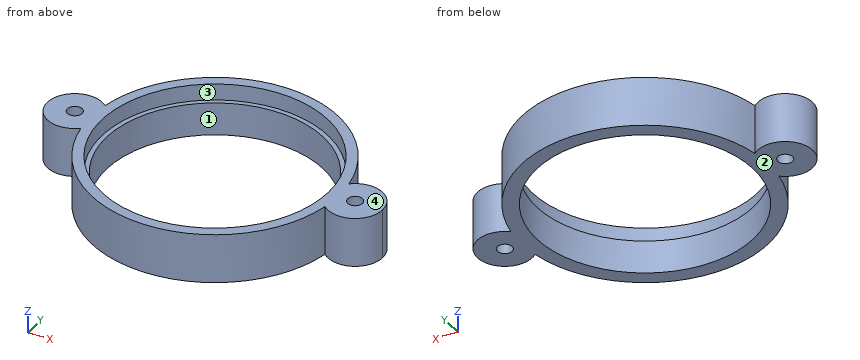
```python
from build123d import *

# Parameters (mm, degrees)
F0_R     = 1.35
F1_DEPTH = 9
F0_R_2   = 19.75
F2_DEPTH = 6
F3_R     = 22.5
F3_R_2   = 20.6
F4_DEPTH = 3


with BuildPart() as f1:
    # F0 (on Top) → F1 (new body)
    with BuildSketch(Plane.XY):
        with BuildLine():
            ThreePointArc((-22.1862745098, -3.7442253372), (-22.5, 0), (-22.1862745098, 3.7442253372))
            ThreePointArc((-22.1862745098, 3.7442253372), (-30.5, 0), (-22.1862745098, -3.7442253372))
        make_face()
        with Locations((-25.5, 0)):
            Circle(F0_R, mode=Mode.SUBTRACT)
    extrude(amount=F1_DEPTH)



with BuildPart() as f1b:
    # F0 (on Top) → F1, piece 2 (new body)
    with BuildSketch(Plane.XY):
        with BuildLine():
            ThreePointArc((22.1862745098, 3.7442253372), (22.4214314493, 1.8786728733), (22.5, 0))
            ThreePointArc((22.5, 0), (22.4214314493, -1.8786728733), (22.1862745098, -3.7442253372))
            ThreePointArc((22.1862745098, -3.7442253372), (27.5532136456, -4.5589816544), (30.5, 0))
            ThreePointArc((30.5, 0), (27.5532136456, 4.5589816544), (22.1862745098, 3.7442253372))
        make_face()
        with Locations((25.5, 0)):
            Circle(F0_R, mode=Mode.SUBTRACT)
    extrude(amount=F1_DEPTH)


with BuildPart() as f2:
    # F0 (on Top) → F2 (new body)
    with BuildSketch(Plane.XY):
        with BuildLine():
            ThreePointArc((22.1862745098, -3.7442253372), (20.5, 0), (22.1862745098, 3.7442253372))
            ThreePointArc((22.1862745098, 3.7442253372), (0, 22.5), (-22.1862745098, 3.7442253372))
            ThreePointArc((-22.1862745098, 3.7442253372), (-20.9410183456, 2.0532136456), (-20.5, 0))
            ThreePointArc((-20.5, 0), (-20.9410183456, -2.0532136456), (-22.1862745098, -3.7442253372))
            ThreePointArc((-22.1862745098, -3.7442253372), (0, -22.5), (22.1862745098, -3.7442253372))
        make_face()
        Circle(F0_R_2, mode=Mode.SUBTRACT)
        with BuildLine():
            ThreePointArc((22.1862745098, -3.7442253372), (22.4214314493, -1.8786728733), (22.5, 0))
            ThreePointArc((22.5, 0), (22.4214314493, 1.8786728733), (22.1862745098, 3.7442253372))
            ThreePointArc((22.1862745098, 3.7442253372), (20.5, 0), (22.1862745098, -3.7442253372))
        make_face()
        with BuildLine():
            ThreePointArc((-20.5, 0), (-20.9410183456, 2.0532136456), (-22.1862745098, 3.7442253372))
            ThreePointArc((-22.1862745098, 3.7442253372), (-22.5, 0), (-22.1862745098, -3.7442253372))
            ThreePointArc((-22.1862745098, -3.7442253372), (-20.9410183456, -2.0532136456), (-20.5, 0))
        make_face()
    extrude(amount=F2_DEPTH)


with BuildPart() as f1_1:
    add(f1.part)

    add(f1b.part)  # F4 merges F1b

    add(f2.part)  # F4 merges F2
    # F3 (on face) → F4 (join)
    with BuildSketch(Plane.XY.offset(6)):
        Circle(F3_R)
        Circle(F3_R_2, mode=Mode.SUBTRACT)
    extrude(amount=F4_DEPTH)


solid = f1_1.part
```
Build history of the part. All positions in model axes, mm. Face numbers are marked on the shaded views. A direction names the side the tool comes from. Round coordinates to 2 decimals unless told otherwise and drop trailing zeros. Loops run counter-clockwise (first coordinate to the right, second up) from the corner with the lowest first, then second, coordinate; pieces in that order, holes last. Notation, with made-up numbers: M 25,-35 L 45,-35 A20 cw 45,-8 Z; hole C -22.5,57.5 d4. An arc over 180 degrees is marked long. Answer as CSV lines item,"result".
1. Cut at B-B on z = 4.25. Write the cut outline in (x, y), then the cut area to 3 significant figures.
Resolved:
outline,"M -22.19,-3.74 A22.5 ccw 22.19,-3.74 A5 ccw long 22.19,3.74 A22.5 ccw -22.19,3.74 A5 ccw long Z; hole C -25.5,0 d2.7; hole C 0,0 d39.5; hole C 25.5,0 d2.7"
area,"490 mm²"
2. Cut at D-D on x = 0. Write the cut outline in (y, z).
Resolved:
outline,"M -22.5,0 L -19.75,0 L -19.75,6 L -20.6,6 L -20.6,9 L -22.5,9 Z; M 19.75,0 L 22.5,0 L 22.5,9 L 20.6,9 L 20.6,6 L 19.75,6 Z"
3. Cut at C-C on y = -14. Write the cut outline in (x, z), then the cut area to 3 significant figures.
Resolved:
outline,"M -17.61,0 L -13.93,0 L -13.93,6 L -15.11,6 L -15.11,9 L -17.61,9 Z; M 13.93,0 L 17.61,0 L 17.61,9 L 15.11,9 L 15.11,6 L 13.93,6 Z"
area,"59.2 mm²"
4. Flat gauge pins, fed straight in: P1, Ø1, axis at y = -10, z = 3, coming from the +X side; P2, Ø4, axis at x = 9, y = -16, coming from the +Z side; P3, Ø1, axis at x = -12, z = 5, coming from the -Y side; P4, Ø2.5, axis at x = 25.5, y = 0, coming from the +Z side. Where does each tip first touch, or does it go through?
Resolved:
P1,"stops at x = 20.4"
P2,"stops at z = 6"
P3,"stops at y = -19.34"
P4,"passes through"
5. 3-axis set-ups, long thin cutter, end or side, ignore diameter. For the marked faces 3 and 4: which of +Z, -Z, +X, -X, +Y, -Y reach the whole face in a straight line?
Resolved:
face 3,"+Z"
face 4,"+Z, +X, -X, +Y, -Y"
6. Cut at A-A on x = 25.5. Write the cut outline in (y, z), then the cut area to 3 significant figures.
Resolved:
outline,"M -5,0 L -1.35,0 L -1.35,9 L -5,9 Z; M 1.35,0 L 5,0 L 5,9 L 1.35,9 Z"
area,"65.7 mm²"
7. Wall check: probe 1 along X at (y, z) = (4, 7.5); probe 2 along Y at (x, z) = (25.5, 3); probe 3 along Y at (x, z) = (0, 2.05). Give the ranges that are in metal, low to high. Write a range as [from, to].
Resolved:
probe 1,"x = [-28.5, -22.5], [-22.14, -20.21], [20.21, 22.14], [22.5, 28.5]"
probe 2,"y = [-5, -1.35], [1.35, 5]"
probe 3,"y = [-22.5, -19.75], [19.75, 22.5]"
8. Two-plate mould, pull along Y, no slides. Class the marked faces 1 and 2: released by +Y, released by -Y, zero draft, split by the parting line, or undercut.
Resolved:
face 1,"undercut"
face 2,"zero draft"
